from build123d import *
from build123d.topology import SkipClean

# Parameters (mm, degrees)
SKETCH1_R           = 76.2
BOSS_EXTRUDE1_DEPTH = 3.81
BOSS_EXTRUDE3_DEPTH = 3.81
SKETCH5_R           = 6.35
CUT_EXTRUDE1_DEPTH  = 212.070408513
BOSS_EXTRUDE4_START = -3.81
BOSS_EXTRUDE4_DEPTH = 16.51
SKETCH8_R           = 3.175
CUT_EXTRUDE3_DEPTH  = 332.331209118
CIRPATTERN3_COUNT   = 4
SKETCH9_R           = 3.174999999
CUT_EXTRUDE4_DEPTH  = 3.81
SKETCH11_R          = 31.75
SKETCH11_R_2        = 25.4
BOSS_EXTRUDE5_DEPTH = 3.81
SKETCH12_R          = 25.4
CUT_EXTRUDE5_DEPTH  = 3.81
SKETCH13_R          = 20.52955
SKETCH13_R_2        = 2.3622
BOSS_EXTRUDE7_DEPTH = 3.81
SKETCH14_R          = 2.3622
CUT_EXTRUDE6_DEPTH  = 3.81
SKETCH15_R          = 3.175
CUT_EXTRUDE7_DEPTH  = 3.81
SKETCH16_R          = 25.4
SKETCH16_R_2        = 18.796
BOSS_EXTRUDE8_DEPTH = 3.81
SKETCH17_R          = 3.175
CUT_EXTRUDE8_DEPTH  = 212.417812192
BOSS_EXTRUDE9_START = -3.81
SKETCH19_R          = 3.175
SKETCH19_R_2        = 2.3622
SKETCH19_R_3        = 3.174999999
BOSS_EXTRUDE9_DEPTH = 3.81


with BuildPart() as part:
    # Sketch1 → Boss-Extrude1 (new body)
    with BuildSketch(Plane(origin=(0, 0, 0), x_dir=(1, 0, 0), z_dir=(0, 1, 0))):
        with Locations(Location((0, 0, 0), (0, 0, 90))):
            Circle(SKETCH1_R)
    extrude(amount=BOSS_EXTRUDE1_DEPTH)

    # Sketch3 → Boss-Extrude3 (add)
    with BuildSketch(Plane(origin=(0, 0, 0), x_dir=(-1, 0, 0), z_dir=(0, -1, 0))):
        with BuildLine():
            Line((9.525, -9.525), (148.920700374, -9.525))
            ThreePointArc((148.920700374, -9.525), (149.225, 0), (148.920700374, 9.525))
            Line((148.920700374, 9.525), (9.525, 9.525))
            Line((9.525, 9.525), (9.525, 148.920700374))
            ThreePointArc((9.525, 148.920700374), (0, 149.225), (-9.525, 148.920700374))
            Line((-9.525, 148.920700374), (-9.525, 9.525))
            Line((-9.525, 9.525), (-148.920700374, 9.525))
            ThreePointArc((-148.920700374, 9.525), (-149.225, 0), (-148.920700374, -9.525))
            Line((-148.920700374, -9.525), (-9.525, -9.525))
            Line((-9.525, -9.525), (-9.525, -148.920700374))
            ThreePointArc((-9.525, -148.920700374), (0, -149.225), (9.525, -148.920700374))
            Line((9.525, -148.920700374), (9.525, -9.525))
        make_face()
    extrude(amount=-BOSS_EXTRUDE3_DEPTH)

    # Sketch5 → Cut-Extrude1 (cut, through all)
    with BuildSketch(Plane(origin=(0, 3.81, 0), x_dir=(1, 0, 0), z_dir=(0, 1, 0))):
        with Locations(Location((0, 0, 0), (0, 0, 270))):
            Circle(SKETCH5_R)
    extrude(amount=-CUT_EXTRUDE1_DEPTH, mode=Mode.SUBTRACT)

    # Sketch7 → Boss-Extrude4 (add)
    with BuildSketch(Plane(origin=(0, 3.81, 0), x_dir=(1, 0, 0), z_dir=(0, 1, 0)).offset(BOSS_EXTRUDE4_START)):
        with BuildLine():
            Line((18.739703318, 148.043656212), (18.739703318, 146.138656212))
            Line((18.739703318, 146.138656212), (-18.739703318, 146.138656212))
            Line((-18.739703318, 146.138656212), (-18.739703318, 148.043656212))
            ThreePointArc((-18.739703318, 148.043656212), (0, 149.225), (18.739703318, 148.043656212))
        make_face()
    boss_extrude4 = extrude(amount=BOSS_EXTRUDE4_DEPTH)

    # Sketch8 → Cut-Extrude3 (cut, through all)
    with BuildSketch(Plane.XY.offset(-146.138656212)):
        with Locations((-9.369851659, 8.255)):
            Circle(SKETCH8_R)
        with Locations((9.369851659, 8.255)):
            Circle(SKETCH8_R)
    cut_extrude3 = extrude(amount=-CUT_EXTRUDE3_DEPTH, mode=Mode.SUBTRACT)

    # CirPattern3: Boss-Extrude4, Cut-Extrude3 ×4 about axis
    cirpattern3_axis = Axis((0, 0, 0), (0, 1, 0))
    add([boss_extrude4.rotate(cirpattern3_axis, i * 360 / CIRPATTERN3_COUNT) for i in range(1, CIRPATTERN3_COUNT)])
    add([cut_extrude3.rotate(cirpattern3_axis, i * 360 / CIRPATTERN3_COUNT) for i in range(1, CIRPATTERN3_COUNT)], mode=Mode.SUBTRACT)

    # Sketch9 → Cut-Extrude4 (cut)
    with BuildSketch(Plane.XZ):
        with Locations(Location((-56.514999999, -23.8125, 0), (0, 0, 270))):
            Circle(SKETCH9_R)
        with Locations(Location((-15.874999999, -23.8125, 0), (0, 0, 270))):
            Circle(SKETCH9_R)
    extrude(amount=-CUT_EXTRUDE4_DEPTH, mode=Mode.SUBTRACT)

    # Sketch11 → Boss-Extrude5 (add)
    with BuildSketch(Plane(origin=(0, 3.81, 0), x_dir=(1, 0, 0), z_dir=(0, 1, 0))):
        with Locations((41.275, -41.275)):
            Circle(SKETCH11_R)
        with Locations((41.275, -41.275)):
            Circle(SKETCH11_R_2, mode=Mode.SUBTRACT)
    extrude(amount=-BOSS_EXTRUDE5_DEPTH)

    # Sketch12 → Cut-Extrude5 (cut)
    with BuildSketch(Plane(origin=(0, 3.81, 0), x_dir=(1, 0, 0), z_dir=(0, 1, 0))):
        with Locations(Location((41.275, -41.275, 0), (0, 0, 270))):
            Circle(SKETCH12_R)
    extrude(amount=-CUT_EXTRUDE5_DEPTH, mode=Mode.SUBTRACT)

    # Sketch13 → Boss-Extrude7 (add)
    with BuildSketch(Plane(origin=(0, 3.81, 0), x_dir=(1, 0, 0), z_dir=(0, 1, 0))):
        with Locations((-41.16870274, -55.03340443)):
            Circle(SKETCH13_R)
        with Locations(Location((-41.17109409, -70.730891948, 0), (0, 0, 270))):
            Circle(SKETCH13_R_2, mode=Mode.SUBTRACT)
        with Locations((-41.166311391, -39.335916913)):
            Circle(SKETCH13_R_2, mode=Mode.SUBTRACT)
    extrude(amount=-BOSS_EXTRUDE7_DEPTH)

    # Sketch14 → Cut-Extrude6 (cut)
    with BuildSketch(Plane(origin=(0, 3.81, 0), x_dir=(1, 0, 0), z_dir=(0, 1, 0))):
        with Locations(Location((-41.166311391, -39.335916913, 0), (0, 0, 270))):
            Circle(SKETCH14_R)
    extrude(amount=-CUT_EXTRUDE6_DEPTH, mode=Mode.SUBTRACT)

    # Sketch15 → Cut-Extrude7 (cut)
    with BuildSketch(Plane(origin=(0, 3.81, 0), x_dir=(1, 0, 0), z_dir=(0, 1, 0))):
        with Locations(Location((16.720717023, -16.720717023, 0), (0, 0, 270))):
            Circle(SKETCH15_R)
        with Locations(Location((65.829282977, -16.720717023, 0), (0, 0, 270))):
            Circle(SKETCH15_R)
        with Locations(Location((16.720717023, -65.829282977, 0), (0, 0, 270))):
            Circle(SKETCH15_R)
    extrude(amount=-CUT_EXTRUDE7_DEPTH, mode=Mode.SUBTRACT)

    # Sketch16 → Boss-Extrude8 (add)
    with BuildSketch(Plane(origin=(0, 3.81, 0), x_dir=(1, 0, 0), z_dir=(0, 1, 0))):
        with Locations((41.275, -41.275)):
            Circle(SKETCH16_R)
        with Locations(Location((41.275, -41.275, 0), (0, 0, 270))):
            Circle(SKETCH16_R_2, mode=Mode.SUBTRACT)
    extrude(amount=-BOSS_EXTRUDE8_DEPTH)

    # Sketch17 → Cut-Extrude8 (cut, through all)
    with BuildSketch(Plane(origin=(0, 3.81, 0), x_dir=(1, 0, 0), z_dir=(0, 1, 0))):
        with BuildLine():
            ThreePointArc((24.172548233, -49.072163558), (22.778717915, -37.931773261), (27.984220941, -27.984220941))
            Line((27.984220941, -27.984220941), (18.965781054, -18.965781054))
            ThreePointArc((18.965781054, -18.965781054), (18.376181742, -19.429971822), (17.694108713, -19.742824503))
            ThreePointArc((17.694108713, -19.742824503), (13.616121159, -36.023762469), (24.172548233, -49.072163558))
        make_face()
        with BuildLine():
            Line((18.965781054, -18.965781054), (27.984220941, -27.984220941))
            ThreePointArc((27.984220941, -27.984220941), (34.167406023, -23.874663111), (41.459517866, -22.479905716))
            Line((41.459517866, -22.479905716), (45.26049085, -18.678932732))
            ThreePointArc((45.26049085, -18.678932732), (32.694581443, -13.187694328), (19.742824503, -17.694108713))
            ThreePointArc((19.742824503, -17.694108713), (19.429971822, -18.376181742), (18.965781054, -18.965781054))
        make_face()
        with Locations(Location((56.523994768, -7.415428814, 0), (0, 0, 270))):
            Circle(SKETCH17_R)
        with Locations(Location((7.415428814, -56.523994768, 0), (0, 0, 270))):
            Circle(SKETCH17_R)
    extrude(amount=-CUT_EXTRUDE8_DEPTH, mode=Mode.SUBTRACT)

    # Sketch19 → Boss-Extrude9 (add)
    with SkipClean():  # the faces are left unmerged after this step: merging them gives an invalid solid
        with BuildSketch(Plane(origin=(0, 3.81, 0), x_dir=(1, 0, 0), z_dir=(0, 1, 0)).offset(BOSS_EXTRUDE9_START)):
            with BuildLine():
                ThreePointArc((24.172548233, -49.072163558), (34.587447779, -58.841054232), (48.86207293, -58.471683993))
                ThreePointArc((48.86207293, -58.471683993), (53.881536726, -53.881536726), (58.471683993, -48.86207293))
                ThreePointArc((58.471683993, -48.86207293), (58.841054232, -34.587447779), (49.072163558, -24.172548233))
                ThreePointArc((49.072163558, -24.172548233), (45.26049085, -45.26049085), (24.172548233, -49.072163558))
            make_face()
            with Locations((65.829282977, -16.720717023)):
                Circle(SKETCH19_R)
            with Locations((16.720717023, -65.829282977)):
                Circle(SKETCH19_R)
            with Locations((-41.17109409, -70.730891948)):
                Circle(SKETCH19_R_2)
            with Locations((-41.166311391, -39.335916913)):
                Circle(SKETCH19_R_2)
            with Locations((-15.874999999, 23.8125)):
                Circle(SKETCH19_R_3)
            with Locations((-56.514999999, 23.8125)):
                Circle(SKETCH19_R_3)
        extrude(amount=BOSS_EXTRUDE9_DEPTH)


solid = part.part
Could you check a few things on this model? Use its own coordinates, in mm. Give positions to 0.01 mm unless a question says otherwise; leave off trailing zeros. Write each loop counter-clockwise with the first axis right and the second up, starting at its lowest first coordinate (ties: lowest second). Pieces come first, ordered by that corner, then holes. Notation, with made-up numbers: (24, 43.25) -> (46, 43.25) arc R23 ccw to (46, 79.25) -> close; hole circle Ø7 at (17.5, 25.25). An arc over 180 degrees is marked (long way). Answer as a JSON object with one key per item and string values.
Q1. Suppose I cut it at C-C on z = 104.5. Write out the boundary of the cut face in (x, y) (3 decimals).
Taken from the geometry:
{"outline": "(-9.525, 0) -> (9.525, 0) -> (9.525, 3.81) -> (-9.525, 3.81) -> close"}
Q2. Please list where these lines run through material, in increasing order: L1, parallel to Y at x = 10, z = -53.5; L2, parallel to X at y = 1.25, z = -137 (3 decimals); L3, parallel to Z at x = -13, y = 4.
Taken from the geometry:
{"L1": "y = 0 to 3.81", "L2": "x = -9.525 to 9.525", "L3": "z = -148.66 to -146.14, 146.14 to 148.66"}
Q3. Suppose I cut it at D-D on z = 41.5. Write out the boundary of the cut face in (x, y).
Taken from the geometry:
{"outline": "(-63.91, 0) -> (15.77, 0) -> (15.77, 3.81) -> (-63.91, 3.81) -> close; (48.17, 0) -> (73.02, 0) -> (73.02, 3.81) -> (48.17, 3.81) -> close"}
Q4. Will these pins go through, and if not, where does the flat tip stop? pin 1 Ø4 at (x, z) = (56.52, 7.42) entering from +Y; pin 2 Ø1.1 at (y, z) = (1, 111.5) entering from -X (3 decimals); pin 3 Ø3 at (x, y) = (20, 11.5) entering from +Z; pin 4 Ø1.9 at (x, y) = (112.5, 1.5) entering from +Z (3 decimals).
Taken from the geometry:
{"pin 1": "passes through", "pin 2": "stops at x = -9.525", "pin 3": "stops at z = 148.07", "pin 4": "stops at z = 9.525"}
Q5. Suppose I cut it at B-B on z = 0. Write out the boundary of the cut face in (x, y) (3 decimals).
Taken from the geometry:
{"outline": "(-149.225, 0) -> (-6.35, 0) -> (-6.35, 3.81) -> (-146.139, 3.81) -> (-146.139, 16.51) -> (-149.225, 16.51) -> close; (6.35, 0) -> (149.225, 0) -> (149.225, 16.51) -> (146.139, 16.51) -> (146.139, 3.81) -> (6.35, 3.81) -> close"}
Q6. We'd pull the mould along X, two halves only. Please class faces 1 (the cylindrical face through (-70.459, 1.878, 29.017)), 2 (the cylindrical face through (14.561, 1.932, 14.393)), 3 (the flat face through (0, 10, -146.139)): released by +X, released by -X, zero draft, split by the parting line, or undercut.
Taken from the geometry:
{"face 1": "undercut", "face 2": "undercut", "face 3": "zero draft"}
Q7. Suppose I cut it at A-A on x = 0. Write out the boundary of the cut face in (y, z) (3 decimals), then the cut area to 3 significant figures.
Taken from the geometry:
{"outline": "(0, -149.225) -> (16.51, -149.225) -> (16.51, -146.139) -> (3.81, -146.139) -> (3.81, -6.35) -> (0, -6.35) -> close; (0, 6.35) -> (3.81, 6.35) -> (3.81, 146.139) -> (16.51, 146.139) -> (16.51, 149.225) -> (0, 149.225) -> close", "area": "1,170 mm²"}
